```python
from build123d import *

# Parameters (mm, degrees)
F1_DEPTH = 50.8
F2_W     = 152.4
F2_H     = 19.05
F3_DEPTH = 3.175


with BuildPart() as f1:
    # F0 (on Front) → F1 (new body)
    with BuildSketch(Plane.XZ):
        Polygon((958.85, 387.35), (704.85, 590.55), (-704.85, 590.55), (-958.85, 387.35), (-958.85, -590.55), (-908.05, -590.55), (-908.05, 362.934258), (-687.030322, 539.75), (687.030322, 539.75), (908.05, 362.934258), (908.05, -590.55), (958.85, -590.55), align=None)
    extrude(amount=F1_DEPTH)

    # F2 (on face) → F3 (cut)
    with BuildSketch(Plane.XZ.offset(50.8)):
        with Locations((-101.6, 565.15)):
            Rectangle(F2_W, F2_H)
        with Locations((101.6, 565.15)):
            Rectangle(F2_W, F2_H)
    extrude(amount=-F3_DEPTH, mode=Mode.SUBTRACT)


solid = f1.part
```
Can you work these out from the model? Positions are in its coordinate system, mm. A direction names the side the tool comes from. Round coordinates to 2 decimals unless told otherwise and drop trailing zeros. Loops run counter-clockwise (first coordinate to the right, second up) from the corner with the lowest first, then second, coordinate; pieces in that order, holes last. Notation, with made-up numbers: (-29, -6) -> (-1, -6) arc R20 ccw to (-1, 20) -> close; hole circle Ø2 at (83.25, 53.5). An arc over 180 degrees is marked (long way). One line per item, written item: value. Start each with the question number.
1. If we mould it in two halves opening along X, with no side actions, what happens to faces 3 (the flat face through (958.85, -25, -108)), 4 (the flat face through (-10, -25, 539.75)), 5 (the flat face through (-958.85, -25, -95)), 6 (the flat face through (-934, -25, -590.55))? For each: pulls with the +X half, pulls with the -X half, needs draft (parallel to the pull), parting line crosses it, or undercut.
2. For pin 1 (3.5 mm diameter, centred on x = 138, y = -49.5, fed in from -Z); pin 2 (9.5 mm diameter, centred on x = 81.5, z = 560.5, fed in from -Y) (3 decimals); pin 3 (1.5 mm diameter, centred on x = 761, y = -20.5, fed in from +Z), each with a flat end and sliding along its axis, tell me the tip position at first contact or that it passes through.
3. If we section it at D-D, the plane z = 518.5: Write out the boundary of the cut face in (x, y), then the cut area to 3 significant figures.
4. If we section it at B-B, the plane y = -24: Write out the boundary of the cut face in (x, z).
5. If we section it at C-C, the plane x = -44.5: Write out the boundary of the cut face in (y, z) (3 decimals), then the cut area to 3 significant figures.
6. If we section it at A-A, the plane z = -60: Write out the boundary of the cut face in (x, y).
7. For faces 1 (the flat face through (795.99, -25.04, 452.58)), 2 (the flat face through (-4, -50.8, 571)), which set-ups out of +Z, -Z, +X, -X, +Y, -Y let a thin tool reach every point of the face, with its end or its side?
8. If I drill on probe 1 along X at (y, z) = (-31.5, -117); probe 2 along Z at (x, y) = (-26.5, -43); probe 3 along X at (y, z) = (-16, 504.5), over which ranges is the centre line in solid material (lowest first)?
Calculated:
1. face 3: pulls with the +X half
1. face 4: undercut
1. face 5: pulls with the -X half
1. face 6: needs draft
2. pin 1: stops at z = 539.75
2. pin 2: stops at y = -47.625
2. pin 3: stops at z = 546.23
3. outline: (-794.91, -50.8) -> (-713.59, -50.8) -> (-713.59, 0) -> (-794.91, 0) -> close; (713.59, -50.8) -> (794.91, -50.8) -> (794.91, 0) -> (713.59, 0) -> close
3. area: 8,260 mm²
4. outline: (-958.85, -590.55) -> (-908.05, -590.55) -> (-908.05, 362.93) -> (-687.03, 539.75) -> (687.03, 539.75) -> (908.05, 362.93) -> (908.05, -590.55) -> (958.85, -590.55) -> (958.85, 387.35) -> (704.85, 590.55) -> (-704.85, 590.55) -> (-958.85, 387.35) -> close
5. outline: (-50.8, 539.75) -> (0, 539.75) -> (0, 590.55) -> (-50.8, 590.55) -> (-50.8, 574.675) -> (-47.625, 574.675) -> (-47.625, 555.625) -> (-50.8, 555.625) -> close
5. area: 2,520 mm²
6. outline: (-958.85, -50.8) -> (-908.05, -50.8) -> (-908.05, 0) -> (-958.85, 0) -> close; (908.05, -50.8) -> (958.85, -50.8) -> (958.85, 0) -> (908.05, 0) -> close
7. face 1: -Z, +Y, -Y
7. face 2: +Z, -Z, +X, -X, -Y
8. probe 1: x = -958.85 to -908.05, 908.05 to 958.85
8. probe 2: z = 539.75 to 590.55
8. probe 3: x = -812.41 to -731.09, 731.09 to 812.41
